from build123d import *

# Parameters (mm, degrees)
F0_R     = 14.2875
F0_R_2   = 3.373438
F1_DEPTH = 2.286


with BuildPart() as f1:
    # F0 (on Right) → F1 (new body)
    with BuildSketch(Plane.YZ):
        with BuildLine():
            ThreePointArc((-41.678018, -70.096295), (-34.493562, -69.059045), (-27.895884, -66.032011))
            Line((-27.895884, -66.032011), (126.930524, 33.980489))
            ThreePointArc((126.930524, 33.980489), (137.51114, 62.500661), (113.14839, 80.716205))
            Line((113.14839, 80.716205), (28.638652, 80.716205))
            ThreePointArc((28.638652, 80.716205), (18.351058, 82.892825), (9.826628, 89.049637))
            Line((9.826628, 89.049637), (-22.94285, 114.364516))
            ThreePointArc((-22.94285, 114.364516), (-42.076779, 119.406552), (-59.022421, 109.190164))
            Line((-59.022421, 109.190164), (-122.859185, 38.763636))
            ThreePointArc((-122.859185, 38.763636), (-127.737616, 30.847053), (-129.439808, 21.705176))
            Line((-129.439808, 21.705176), (-129.439808, -44.696295))
            ThreePointArc((-129.439808, -44.696295), (-122.000321, -62.656807), (-104.039808, -70.096295))
            Line((-104.039808, -70.096295), (-41.678018, -70.096295))
        make_face()
        Polygon((-85.084374, -52.344054), (-97.784249, -52.287691), (-104.085375, -41.261095), (-97.686626, -30.290862), (-84.986751, -30.347225), (-78.685625, -41.373821), align=None, mode=Mode.SUBTRACT)
        Polygon((-57.446231, -38.402657), (-70.146106, -38.346295), (-76.447232, -27.319699), (-70.048483, -16.349466), (-57.348608, -16.405829), (-51.047482, -27.432424), align=None, mode=Mode.SUBTRACT)
        with Locations((-29.411834, -38.346295)):
            Circle(F0_R, mode=Mode.SUBTRACT)
        Polygon((-85.096416, -23.010039), (-97.796291, -22.953676), (-104.097417, -11.927081), (-97.698668, -0.956848), (-84.998793, -1.01321), (-78.697667, -12.039806), align=None, mode=Mode.SUBTRACT)
        Polygon((-57.543857, -7.94989), (-70.243732, -7.893527), (-76.544858, 3.133069), (-70.146109, 14.103302), (-57.446234, 14.046939), (-51.145108, 3.020343), align=None, mode=Mode.SUBTRACT)
        Polygon((-85.038808, 5.336948), (-97.738683, 5.393311), (-104.039808, 16.419906), (-97.641059, 27.390139), (-84.941185, 27.333776), (-78.640059, 16.307181), align=None, mode=Mode.SUBTRACT)
        Polygon((-28.643053, 9.313772), (-41.342928, 9.370135), (-47.644054, 20.396731), (-41.245305, 31.366964), (-28.54543, 31.310601), (-22.244304, 20.284005), align=None, mode=Mode.SUBTRACT)
        Polygon((-2.817801, -5.711303), (-15.517676, -5.65494), (-21.818802, 5.371655), (-15.420052, 16.341888), (-2.720178, 16.285526), (3.580948, 5.25893), align=None, mode=Mode.SUBTRACT)
        Polygon((22.526503, -18.976484), (9.826628, -18.920122), (3.525502, -7.893526), (9.924251, 3.076707), (22.624126, 3.020344), (28.925252, -8.006251), align=None, mode=Mode.SUBTRACT)
        Polygon((22.371272, 9.370136), (9.671397, 9.426499), (3.370271, 20.453094), (9.76902, 31.423327), (22.468895, 31.366965), (28.770021, 20.340369), align=None, mode=Mode.SUBTRACT)
        Polygon((48.145067, -5.711305), (35.445192, -5.654942), (29.144066, 5.371654), (35.542815, 16.341887), (48.24269, 16.285524), (54.543816, 5.258928), align=None, mode=Mode.SUBTRACT)
        Polygon((73.847689, 10.850061), (61.147815, 10.906608), (54.84685, 21.933296), (61.245758, 32.903436), (73.945632, 32.846888), (80.246598, 21.820201), align=None, mode=Mode.SUBTRACT)
        Polygon((-57.699089, 20.396731), (-70.398963, 20.453093), (-76.700089, 31.479689), (-70.30134, 42.449922), (-57.601465, 42.393559), (-51.30034, 31.366964), align=None, mode=Mode.SUBTRACT)
        Polygon((-57.641481, 48.743717), (-70.341355, 48.80008), (-76.642481, 59.826676), (-70.243732, 70.796909), (-57.543857, 70.740546), (-51.242732, 59.71395), align=None, mode=Mode.SUBTRACT)
        Polygon((-2.973032, 22.635317), (-15.672907, 22.69168), (-21.974033, 33.718276), (-15.575284, 44.688509), (-2.875409, 44.632146), (3.425717, 33.60555), align=None, mode=Mode.SUBTRACT)
        with Locations((-37.046294, 56.249909)):
            Circle(F0_R_2, mode=Mode.SUBTRACT)
        Polygon((-2.915424, 50.982304), (-15.615299, 51.038667), (-21.916425, 62.065262), (-15.517676, 73.035495), (-2.817801, 72.979133), (3.483325, 61.952537), align=None, mode=Mode.SUBTRACT)
        with Locations((-37.046294, 81.649909)):
            Circle(F0_R, mode=Mode.SUBTRACT)
        with Locations((-37.046294, 107.049909)):
            Circle(F0_R_2, mode=Mode.SUBTRACT)
        Polygon((47.989836, 22.635315), (35.289961, 22.691678), (28.988835, 33.718274), (35.387584, 44.688507), (48.087459, 44.632144), (54.388585, 33.605548), align=None, mode=Mode.SUBTRACT)
        Polygon((22.42888, 37.717123), (9.729005, 37.773485), (3.427879, 48.800081), (9.826628, 59.770314), (22.526503, 59.713951), (28.827629, 48.687356), align=None, mode=Mode.SUBTRACT)
        Polygon((48.047444, 50.982302), (35.347569, 51.038665), (29.046443, 62.065261), (35.445192, 73.035494), (48.145067, 72.979131), (54.446193, 61.952535), align=None, mode=Mode.SUBTRACT)
        with Locations((79.656299, 53.728705)):
            Circle(F0_R, mode=Mode.SUBTRACT)
        with Locations((115.216299, 53.728705)):
            Circle(F0_R, mode=Mode.SUBTRACT)
    extrude(amount=F1_DEPTH)


solid = f1.part
Here's how the part is built. I have some questions about the finished solid (model axes, mm). A direction names the side the tool comes from. Give positions to 0.01 mm unless a question says otherwise; leave off trailing zeros. Loops run counter-clockwise (first coordinate to the right, second up) from the corner with the lowest first, then second, coordinate; pieces in that order, holes last. Notation, with made-up numbers: (34.25, 1.5) -> (65.25, 1.5) arc R14 cw to (65.25, 10.5) -> close; hole circle Ø11 at (-22, -30.75). An arc over 180 degrees is marked (long way). Answer as a JSON object with one key per item and string values. Group by question number.
Item 1: On a 3-axis mill with a long thin cutter (end or side, diameter ignored), from which of +Z, -Z, +X, -X, +Y, -Y can I reach the whole of each face in a straight line? I mean faces 1 (the flat face through (1.13, -81.88, -35.78)), 2 (the flat face through (1.127, -90.494, 74.47)). Say none if no direction works.
Item 2: I need wall thicknesses on L1, parallel to Z at x = 0.15, y = 47.5; L2, parallel to Z at x = 0.2, y = -30; L3, parallel to Y at x = 2.1, z = 31.5. Which ranges of each line are inside material? Lowest first, please.
Item 3: Will this pin go through, and if not, where does the flat tip stop? pin 1 (11 mm diameter, centred on y = -37.05, z = 107.05, fed in from +X).
Item 4: Imagine slicing it at C-C on y = 77. Write out the boundary of the cut face in (x, z).
Item 5: Imagine slicing it at D-D on x = 0.9. Give the number of separate pieces and of enclosed holes in the cut face, then the cut area to 3 significant figures.
Item 6: Imagine slicing it at A-A on z = -35. Write out the boundary of the cut face in (x, y), then the cut area to 3 significant figures.
Item 7: Thinking about a two-plate mould opening in Y: for faces 3 (the flat face through (1.13, 48.43, -16.73)), 4 (the flat face through (1.127, -25.439, 25.874)), 5 (the cylindrical face through (1.127, -122.197, -62.458)), which applies, pulls with the +Y half, pulls with the -Y half, needs draft (parallel to the pull), parting line crosses it, or undercut?
Item 8: Imagine slicing it at B-B on y = 0. Write out the boundary of the cut face in (x, z).
Answer list:
{
 "1": {"face 1": "+X, -X", "face 2": "+Z, +X, -X, -Y"},
 "2": {"L1": "z = -17.33 to -5.71, 16.29 to 22.64, 44.63 to 50.98, 72.98 to 80.72", "L2": "z = -67.25 to -52.62, -24.07 to 9.32, 31.32 to 69.22, 94.08 to 118.21", "L3": "y = -127.48 to -76.69, -51.38 to -20.71, 2.2 to 30.26, 53.16 to 60.43, 74.72 to 123.09"},
 "3": {"pin 1": "stops at x = 2.29"},
 "4": {"outline": "(0, 1.73) -> (2.29, 1.73) -> (2.29, 16.25) -> (0, 16.25) -> close; (0, 27.5) -> (2.29, 27.5) -> (2.29, 39.69) -> (0, 39.69) -> close; (0, 67.77) -> (2.29, 67.77) -> (2.29, 80.72) -> (0, 80.72) -> close"},
 "5": {"separate pieces": "1", "enclosed holes": "24", "area": "21,600 mm2"},
 "6": {"outline": "(0, -129.44) -> (2.29, -129.44) -> (2.29, -100.43) -> (0, -100.43) -> close; (0, -82.33) -> (2.29, -82.33) -> (2.29, -72.06) -> (0, -72.06) -> close; (0, -55.46) -> (2.29, -55.46) -> (2.29, -43.3) -> (0, -43.3) -> close; (0, -15.52) -> (2.29, -15.52) -> (2.29, 20.14) -> (0, 20.14) -> close", "area": "199 mm2"},
 "7": {"face 3": "pulls with the +Y half", "face 4": "undercut", "face 5": "pulls with the -Y half"},
 "8": {"outline": "(0, -48.01) -> (2.29, -48.01) -> (2.29, -0.88) -> (0, -0.88) -> close; (0, 11.53) -> (2.29, 11.53) -> (2.29, 27.73) -> (0, 27.73) -> close; (0, 39.6) -> (2.29, 39.6) -> (2.29, 55.98) -> (0, 55.98) -> close; (0, 68.05) -> (2.29, 68.05) -> (2.29, 96.64) -> (0, 96.64) -> close"}
}
